```python
from build123d import *

# Parameters (mm, degrees)
F0_W      = 63.8407319784
F0_H      = 41.8170765042
F1_DEPTH  = 3.81
F2_R      = 5.08
F3_W      = 63.8407319784
F3_H      = 11.1512206495
F4_DEPTH  = 67.31
F6_DEPTH  = 21.844
F8_D      = 12.7
F9_W      = 18.1207312271
F9_H      = 49.9326833737
F10_DEPTH = 25.4
F12_DEPTH = 25.4


# Not quite as in the source:
# - a feature of the source that left no trace in its solid (it failed there, or was rolled back) is left out


with BuildPart() as f1:
    # F0 (on Top) → F1 (new body)
    with BuildSketch(Plane.XY):
        Rectangle(F0_W, F0_H)
    extrude(amount=F1_DEPTH)

    # F2
    f2_edges = [f1.edges().sort_by_distance(p)[0] for p in [
        (-31.920366, -20.908538, 1.905),
        (31.920366, -20.908538, 1.905),
    ]]
    fillet(f2_edges, radius=F2_R)

    # F3 (on face) → F4 (join)
    with BuildSketch(Plane.XY.offset(3.81)):
        with Locations((0, 15.3329279274)):
            Rectangle(F3_W, F3_H)
    extrude(amount=F4_DEPTH)

    # F5 (on face) → F6 (join)
    with BuildSketch(Plane.XZ.offset(-9.7573176026)):
        with BuildLine():
            ThreePointArc((1.435e-07, 71.12), (-9.6811538885, 47.7476271561), (13.6912190568, 57.4287809432))
            ThreePointArc((13.6912190568, 57.4287809432), (9.6811538885, 67.1099347302), (1.435e-07, 71.12))
        make_face()
    extrude(amount=F6_DEPTH)

    # F8 (through all)
    with Locations(Plane.XZ.offset(12.0866823974)):
        with Locations((0, 57.4287809432)):
            Hole(F8_D / 2)

    # F9 (on face) → F10 (cut)
    with BuildSketch(Plane.XZ.offset(-9.7573176026)):
        with Locations((-22.8600003757, 46.1536583132)):
            Rectangle(F9_W, F9_H)
        with BuildLine():
            Line((13.5208535939, 71.12), (-1.606e-07, 71.12))
            ThreePointArc((-1.606e-07, 71.12), (8.8873621455, 67.8433991962), (13.5208535939, 59.5819175746))
            Line((13.5208535939, 59.5819175746), (13.5208535939, 71.12))
        make_face()
        with BuildLine():
            Line((31.9203659892, 71.12), (13.5208535939, 71.12))
            Line((13.5208535939, 71.12), (13.5208535939, 59.5819175746))
            ThreePointArc((13.5208535939, 59.5819175746), (13.6485612365, 58.5087140134), (13.6912190568, 57.4287809432))
            ThreePointArc((13.6912190568, 57.4287809432), (13.6485612365, 56.3488478729), (13.5208535939, 55.2756443117))
            Line((13.5208535939, 55.2756443117), (13.5208535939, 21.7448789626))
            Line((13.5208535939, 21.7448789626), (31.9203659892, 21.7448789626))
            Line((31.9203659892, 21.7448789626), (31.9203659892, 71.12))
        make_face()
    extrude(amount=-F10_DEPTH, mode=Mode.SUBTRACT)

    # F11 (on face) → F12 (cut)
    with BuildSketch(Plane.XZ.offset(-9.7573176026)):
        with BuildLine():
            ThreePointArc((-29.2383271601, 3.81), (-18.5726517534, 9.7416628621), (-14.3372927251, 21.1873166263))
            Line((-14.3372927251, 21.1873166263), (-31.9203659892, 21.1873166263))
            Line((-31.9203659892, 21.1873166263), (-31.9203659892, 3.81))
            Line((-31.9203659892, 3.81), (-29.2383271601, 3.81))
        make_face()
        with BuildLine():
            ThreePointArc((14.1373165346, 21.7448789626), (19.3458511297, 9.1703641031), (31.9203659892, 3.9618295081))
            Line((31.9203659892, 3.9618295081), (31.9203659892, 21.7448789626))
            Line((31.9203659892, 21.7448789626), (14.1373165346, 21.7448789626))
        make_face()
    extrude(amount=-F12_DEPTH, mode=Mode.SUBTRACT)


solid = f1.part
```
Could you check a few things on this model? Use its own coordinates, in mm. A direction names the side the tool comes from. Give positions to 0.01 mm unless a question says otherwise; leave off trailing zeros. Loops run counter-clockwise (first coordinate to the right, second up) from the corner with the lowest first, then second, coordinate; pieces in that order, holes last. Notation, with made-up numbers: (11, 86) -> (41, 86) arc R28 cw to (41, 113) -> close; hole circle Ø1 at (-33, -12.5). An arc over 180 degrees is marked (long way). Put each result on its own line as item: value.
(1) Thinking about a two-plate mould opening in Z: for faces 4 (the face through (-1, 9.757, 22)), 5 (the face through (5.9, -12.087, 54.6)), 6 (the face through (0, 0, 0)), which applies, pulls with the +Z half, pulls with the -Z half, needs draft (parallel to the pull), parting line crosses it, or undercut?
Computed:
face 4: undercut
face 5: needs draft
face 6: pulls with the -Z half
(2) Imagine slicing it at B-B on x = 1.5. Write out the boundary of the cut face in (y, z).
Computed:
outline: (-20.91, 0) -> (20.91, 0) -> (20.91, 51.26) -> (-12.09, 51.26) -> (-12.09, 43.82) -> (9.76, 43.82) -> (9.76, 3.81) -> (-20.91, 3.81) -> close; (-12.09, 63.6) -> (20.91, 63.6) -> (20.91, 71.04) -> (-12.09, 71.04) -> close
(3) Imagine slicing it at D-D on z = 45.5. Write out the boundary of the cut face in (x, y), plus the area to 3 significant figures.
Computed:
outline: (-13.8, 9.76) -> (-6.72, 9.76) -> (-6.72, -12.09) -> (6.72, -12.09) -> (6.72, 9.76) -> (13.52, 9.76) -> (13.52, 20.91) -> (-13.8, 20.91) -> close
area: 598 mm^2
(4) For faces 1 (the face through (30.39, -19.46, 1.93)), 2 (the face through (-13.8, 15, 46)), 3 (the face through (13.521, 15, 39)), which set-ups out of +Z, -Z, +X, -X, +Y, -Y let a thin tool reach every point of the face, with its end or its side?
Computed:
face 1: +Z, -Z, +X, -Y
face 2: +Z, -X, +Y, -Y
face 3: +X, +Y, -Y
(5) Imagine slicing it at A-A on y = -1.5. Write out the boundary of the cut face in (x, z).
Computed:
outline: (-31.92, 0) -> (31.92, 0) -> (31.92, 3.81) -> (-31.92, 3.81) -> close; circle Ø27.38 at (0, 57.43); hole circle Ø12.7 at (0, 57.43)
(6) Imagine slicing it at C-C on y = 13.5. Write out the boundary of the cut face in (x, z).
Computed:
outline: (-31.92, 0) -> (31.92, 0) -> (31.92, 3.96) arc R17.78 cw to (14.14, 21.74) -> (13.52, 21.74) -> (13.52, 55.28) arc R13.69 ccw to (0, 71.12) -> (-13.8, 71.12) -> (-13.8, 21.19) -> (-14.34, 21.19) arc R17.58 cw to (-29.24, 3.81) -> (-31.92, 3.81) -> close; hole circle Ø12.7 at (0, 57.43)
(7) Please list where these lines run through material, in increasing order: probe 1 along Z at (x, y) = (-0.5, 5); probe 2 along Z at (x, y) = (0, 11.5); probe 3 along Z at (x, y) = (9.5, -19). Write a range as [from, to].
Computed:
probe 1: [0, 3.81], [43.75, 51.1], [63.76, 71.11]
probe 2: [0, 51.08], [63.78, 71.12]
probe 3: [0, 3.81]
(8) I'm going to push flat-ended pins straight in: pin 1 Ø9 at (y, z) = (16, 58.5) entering from -X; pin 2 Ø12.5 at (y, z) = (16, 44.5) entering from +X; pin 3 Ø4 at (y, z) = (15, 14.5) entering from +X; pin 4 Ø12 at (x, z) = (22, 43.5) entering from +Y. Where does each tip first touch, or does it pass through?
Computed:
pin 1: x = -13.8
pin 2: x = 13.52
pin 3: x = 16.73
pin 4: through
